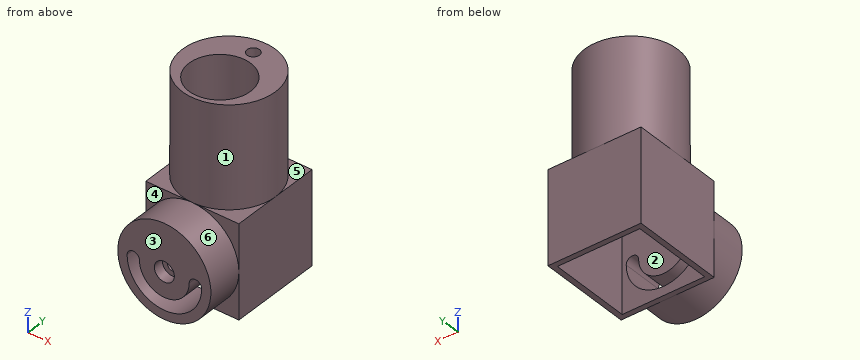
from build123d import *

# Parameters (mm, degrees)
SKETCH1_R           = 28.1
BOSS_EXTRUDE2_DEPTH = 61.3
SKETCH3_R           = 18.6
CUT_EXTRUDE2_DEPTH  = 58.8
SKETCH4_W           = 56.2
SKETCH4_H           = 56.2
BOSS_EXTRUDE3_DEPTH = 56.2
SKETCH5_R           = 16.1
CUT_EXTRUDE4_DEPTH  = 5
SKETCH6_W           = 49.797391422
SKETCH6_H           = 49.779255452
CUT_EXTRUDE5_DEPTH  = 53.7
SKETCH7_R           = 28.1
BOSS_EXTRUDE4_DEPTH = 21.5
CUT_EXTRUDE6_DEPTH  = 21.5
SKETCH9_R           = 3
CUT_EXTRUDE7_DEPTH  = 9.5
SKETCH10_R          = 6.025
CUT_EXTRUDE8_DEPTH  = 6.2
SKETCH18_R          = 3.75
CUT_EXTRUDE9_DEPTH  = 100
SKETCH19_R          = 3.75
CUT_EXTRUDE11_DEPTH = 25


with BuildPart() as part:
    # Sketch1 → Boss-Extrude2 (new body)
    with BuildSketch(Plane.XY):
        Circle(SKETCH1_R)
    extrude(amount=BOSS_EXTRUDE2_DEPTH)

    # Sketch3 → Cut-Extrude2 (cut)
    with BuildSketch(Plane.XY.offset(61.3)):
        with Locations((0, -7)):
            Circle(SKETCH3_R)
    extrude(amount=-CUT_EXTRUDE2_DEPTH, mode=Mode.SUBTRACT)

    # Sketch4 → Boss-Extrude3 (add)
    with BuildSketch(Plane(origin=(0, 0, 0), x_dir=(-1, 0, 0), z_dir=(0, 0, -1))):
        Rectangle(SKETCH4_W, SKETCH4_H)
    extrude(amount=BOSS_EXTRUDE3_DEPTH)

    # Sketch5 → Cut-Extrude4 (cut)
    with BuildSketch(Plane.XY.offset(2.5)):
        with Locations((0, -7)):
            Circle(SKETCH5_R)
    extrude(amount=-CUT_EXTRUDE4_DEPTH, mode=Mode.SUBTRACT)

    # Sketch6 → Cut-Extrude5 (cut)
    with BuildSketch(Plane(origin=(0, 0, -56.2), x_dir=(-1, 0, 0), z_dir=(0, 0, -1))):
        Rectangle(SKETCH6_W, SKETCH6_H)
    extrude(amount=-CUT_EXTRUDE5_DEPTH, mode=Mode.SUBTRACT)

    # Sketch7 → Boss-Extrude4 (add)
    with BuildSketch(Plane(origin=(0, -28.1, 0), x_dir=(-1, 0, 0), z_dir=(0, -1, 0))):
        with Locations(Location((0, 28.1, 0), (0, 0, 90))):
            Circle(SKETCH7_R)
    extrude(amount=BOSS_EXTRUDE4_DEPTH)

    # Sketch8 → Cut-Extrude6 (cut)
    with BuildSketch(Plane(origin=(0, -49.6, 0), x_dir=(-1, 0, 0), z_dir=(0, -1, 0))):
        with BuildLine():
            Line((1.658312395, 25.832078896), (-1.658312395, 25.832078896))
            ThreePointArc((-1.658312395, 25.832078896), (0, 31.332078896), (1.658312395, 25.832078896))
        make_face()
    extrude(amount=-CUT_EXTRUDE6_DEPTH, mode=Mode.SUBTRACT)

    # Sketch9 → Cut-Extrude7 (cut)
    with BuildSketch(Plane(origin=(0, -49.6, 0), x_dir=(-1, 0, 0), z_dir=(0, -1, 0))):
        with Locations(Location((0, 28.332078896, 0), (0, 0, 90))):
            Circle(SKETCH9_R)
    extrude(amount=-CUT_EXTRUDE7_DEPTH, mode=Mode.SUBTRACT)

    # Sketch10 → Cut-Extrude8 (cut)
    with BuildSketch(Plane(origin=(0, -49.6, 0), x_dir=(-1, 0, 0), z_dir=(0, -1, 0))):
        with Locations(Location((0, 28.332078896, 0), (0, 0, 90))):
            Circle(SKETCH10_R)
    extrude(amount=-CUT_EXTRUDE8_DEPTH, mode=Mode.SUBTRACT)

    # Cut-Sweep4: sweep along a path in Sketch15
    with BuildLine(Plane(origin=(0, -49.6, 0), x_dir=(-1, 0, 0), z_dir=(0, -1, 0))) as cut_sweep4_path:
        ThreePointArc((15, 28.332078896), (0, 43.332078896), (-15, 28.332078896))
    # 3DSketch2 → Cut-Sweep4 (sweep, cut)
    with BuildSketch(Plane(origin=(-15, -49.6, -28.332078896), x_dir=(-0.24561664909913958, 0.9693670417779378, 0), z_dir=(0, 0, 1))):
        Polygon((0, 0), (1.842124868, 7.270252813), (30.535389305, 0), (28.693264437, -7.270252813), align=None)
    sweep(path=cut_sweep4_path.line, mode=Mode.SUBTRACT)

    # Sketch18 → Cut-Extrude9 (cut)
    with BuildSketch(Plane.XY.offset(61.3)):
        with Locations((0, 18.75)):
            Circle(SKETCH18_R)
    extrude(amount=-CUT_EXTRUDE9_DEPTH, mode=Mode.SUBTRACT)

    # Sketch19 → Cut-Extrude11 (cut)
    with BuildSketch(Plane(origin=(0, -49.6, 0), x_dir=(-1, 0, 0), z_dir=(0, -1, 0))):
        with Locations((-18.75, 28.332078896)):
            Circle(SKETCH19_R)
        with Locations((18.75, 28.332078896)):
            Circle(SKETCH19_R)
    extrude(amount=-CUT_EXTRUDE11_DEPTH, mode=Mode.SUBTRACT)


solid = part.part
Read the model definition and answer for the solid it produces. Units are mm, in the model's axes. Face numbers are marked on the shaded views. A direction names the side the tool comes from. Round coordinates to 2 decimals unless told otherwise and drop trailing zeros. Order: outer loops, then holes, each group sorted by start corner. A loop starts at its lowest first (then second) coordinate and runs counter-clockwise, first axis right, second up. Notation, with made-up numbers: (-16.5, 15.25) - (-6.5, 15.25) arc R15 cw to (-6.5, 43.25) - close; hole circle Ø10 at (7, 56.25). An arc over 180 degrees is marked (long way). Use one line per item in the form item = value. Start each with the question number.
(1) For the marked faces 4, 5 and 6, determine the directions among +Z, -Z, +X, -X, +Y, -Y from which every point of the face is accessible in a straight line to the end or side of a thin tool.
(2) The part is cut by section B-B (z = -40.5). Give the vertices of the cut face in (x, y), then the cut area to 3 significant figures.
(3) The part is cut by section D-D (y = 18.75). Give the vertices of the cut face in (x, z).
(4) Find the intervals of material crossed by line 1 along Z through (x, y) = (0, -36.25); line 2 along X through (y, z) = (-5, -49.5); line 3 along Y through (x, z) = (22.5, -27), in increasing order. Write a range as from..to.
(5) The part is cut by section C-C (x = 9.5). Give the vertices of the cut face in (y, z), then the cut area to 3 significant figures.
(6) Determine the mould class of the marked faces 1, 2 and 3 for opening direction X: +X half, -X half, draft (parallel to the pull), parting line (faces both ways), or undercut.
(7) The part is cut by section A-A (y = -42). Give the vertices of the cut face in (x, z), then the cut area to 3 significant figures.
(8) Flat-ended cylindrical pins translate along their axes: pin 1 Ø10 at (y, z) = (-7.5, 21.5) entering from +X; pin 2 Ø13.5 at (x, z) = (2, -27) entering from -Y; pin 3 Ø3 at (x, z) = (-12, -1) entering from -Y; pin 4 Ø5 at (x, y) = (20.5, -13) entering from -Z. Find the tip coordinate at first contact, or state that the pin passes through.
Checked values:
q1.face_4 = +Z, -X, -Y
q1.face_5 = +Z, +X, +Y
q1.face_6 = -Y
q2.outline = (-28.1, -28.1) - (-25.22, -28.1) - (-25.22, -49.6) - (-18.93, -49.6) - (-18.93, -24.89) - (-24.9, -24.89) - (-24.9, 24.89) - (24.9, 24.89) - (24.9, -24.89) - (18.93, -24.89) - (18.93, -49.6) - (25.22, -49.6) - (25.22, -28.1) - (28.1, -28.1) - (28.1, 28.1) - (-28.1, 28.1) - close; (-8.77, -49.6) - (8.77, -49.6) - (8.77, -24.89) - (-8.77, -24.89) - close
q2.area = 1,260 mm^2
q3.outline = (-28.1, -56.2) - (-24.9, -56.2) - (-24.9, -2.5) - (-3.75, -2.5) - (-3.75, 61.3) - (-20.93, 61.3) - (-20.93, 0) - (-28.1, 0) - close; (3.75, -2.5) - (24.9, -2.5) - (24.9, -56.2) - (28.1, -56.2) - (28.1, 0) - (20.93, 0) - (20.93, 61.3) - (3.75, 61.3) - close
q4.line_1 = -56.2..-50.83, -43.33..-31.33, -25.83..0
q4.line_2 = -28.1..-24.9, 24.9..28.1
q4.line_3 = -49.6..-24.89, 24.89..28.1
q5.outline = (-49.6, -54.55) - (-28.1, -54.55) - (-28.1, -56.2) - (-24.89, -56.2) - (-24.89, -48.73) - (-49.6, -48.73) - close; (-49.6, -39.94) - (-24.89, -39.94) - (-24.89, -2.5) - (-20, -2.5) - (-20, 2.5) - (-22.99, 2.5) - (-22.99, 61.3) - (-26.45, 61.3) - (-26.45, 0) - (-28.1, 0) - (-28.1, -1.65) - (-49.6, -1.65) - close; (6, -2.5) - (24.89, -2.5) - (24.89, -56.2) - (28.1, -56.2) - (28.1, 0) - (26.45, 0) - (26.45, 61.3) - (8.99, 61.3) - (8.99, 2.5) - (6, 2.5) - close
q5.area = 2,640 mm^2
q6.face_1 = parting line
q6.face_2 = undercut
q6.face_3 = draft
q7.outline = circle Ø56.2 at (0, -28.1); hole (-22.5, -28.33) arc R22.5 ccw to (22.5, -28.33) arc R3.75 ccw to (15, -28.33) arc R15 cw to (-15, -28.33) arc R3.75 ccw to start; hole circle Ø6 at (0, -28.33)
q7.area = 1,970 mm^2
q8.pin_1 = 27.99
q8.pin_2 = -49.6
q8.pin_3 = -28.1
q8.pin_4 = -2.5
